The listing builds one solid part. Answer for the finished solid, in the listing's coordinates (mm). A direction names the side the tool comes from. Give positions to 0.01 mm unless a question says otherwise; leave off trailing zeros. Write each loop counter-clockwise with the first axis right and the second up, starting at its lowest first coordinate (ties: lowest second). Pieces come first, ordered by that corner, then holes. Notation, with made-up numbers: (33.25, 12) -> (79.25, 12) arc R26 cw to (79.25, 44) -> close; hole circle Ø10 at (76.25, 57.25). An arc over 180 degrees is marked (long way). Use CSV: the item, a comma, the result in double quotes. Start each with the question number.
from build123d import *

# Parameters (mm, degrees)
SKETCH1_W           = 114.3
SKETCH1_H           = 177.8
SKETCH1_W_2         = 101.6
SKETCH1_H_2         = 165.1
BOSS_EXTRUDE1_DEPTH = 4.7625
SKETCH2_W           = 12.38677804
SKETCH2_H           = 4.7625
SKETCH2_W_2         = 12.7
BOSS_EXTRUDE2_DEPTH = 4.7625
SKETCH3_W           = 12.7
SKETCH3_H           = 4.7625
BOSS_EXTRUDE3_DEPTH = 4.7625
SKETCH4_W           = 12.7
SKETCH4_H           = 177.8
SKETCH4_W_2         = 3.81
SKETCH4_H_2         = 127
BOSS_EXTRUDE4_DEPTH = 4.7625
FILLET1_R           = 1.905


with BuildPart() as part:
    # Sketch1 → Boss-Extrude1 (new body)
    with BuildSketch(Plane(origin=(0, 0, 0), x_dir=(1, 0, 0), z_dir=(0, 1, 0))):
        Rectangle(SKETCH1_W, SKETCH1_H)
        Rectangle(SKETCH1_W_2, SKETCH1_H_2, mode=Mode.SUBTRACT)
    extrude(amount=BOSS_EXTRUDE1_DEPTH)

    # Sketch2 → Boss-Extrude2 (add)
    with BuildSketch(Plane.XY.offset(88.9)):
        with Locations((-38.1, 2.38125)):
            Rectangle(SKETCH2_W, SKETCH2_H)
        with Locations((12.7, 2.38125)):
            Rectangle(SKETCH2_W_2, SKETCH2_H)
    extrude(amount=BOSS_EXTRUDE2_DEPTH)

    # Sketch3 → Boss-Extrude3 (add)
    with BuildSketch(Plane(origin=(0, 0, -88.9), x_dir=(-1, 0, 0), z_dir=(0, 0, -1))):
        with Locations((-38.1, 2.38125)):
            Rectangle(SKETCH3_W, SKETCH3_H)
        with Locations((12.7, 2.38125)):
            Rectangle(SKETCH3_W, SKETCH3_H)
    extrude(amount=BOSS_EXTRUDE3_DEPTH)

    # Sketch4 → Boss-Extrude4 (add)
    # profile 1 of 2: a face of its own
    with BuildSketch(Plane(origin=(0, 4.7625, 0), x_dir=(-1, 0, 0), z_dir=(0, 1, 0))):
        with Locations((12.7, 0)):
            Rectangle(SKETCH4_W, SKETCH4_H)
        with Locations((12.7, 0)):
            Rectangle(SKETCH4_W_2, SKETCH4_H_2, mode=Mode.SUBTRACT)
    # profile 2 of 2: a face of its own
    with BuildSketch(Plane(origin=(0, 4.7625, 0), x_dir=(-1, 0, 0), z_dir=(0, 1, 0))):
        with Locations((-12.7, 0)):
            Rectangle(SKETCH4_W, SKETCH4_H)
        with Locations((-12.7, 0)):
            Rectangle(SKETCH4_W_2, SKETCH4_H_2, mode=Mode.SUBTRACT)
    extrude(amount=-BOSS_EXTRUDE4_DEPTH)

    # Fillet1
    fillet1_edges = [part.edges().sort_by_distance(p)[0] for p in [
        (-10.795, 2.38125, -63.5),
        (-14.605, 2.38125, -63.5),
        (10.795, 2.38125, -63.5),
        (14.605, 2.38125, -63.5),
        (-10.795, 2.38125, 63.5),
        (-14.605, 2.38125, 63.5),
        (10.795, 2.38125, 63.5),
        (14.605, 2.38125, 63.5),
        (-6.35, 2.38125, 82.55),
        (6.35, 2.38125, 82.55),
        (-6.35, 2.38125, -82.55),
        (6.35, 2.38125, -82.55),
        (-19.05, 2.38125, -82.55),
        (-50.8, 2.38125, -82.55),
        (-50.8, 2.38125, 82.55),
        (-19.05, 2.38125, 82.55),
        (19.05, 2.38125, 82.55),
        (50.8, 2.38125, 82.55),
        (19.05, 2.38125, -82.55),
        (50.8, 2.38125, -82.55),
    ]]
    fillet(fillet1_edges, radius=FILLET1_R - 0.0001)  # a hair under: the kernel refuses the full size


solid = part.part
Q1. Straight lines are drawn through the part: L1, parallel to X at y = 0.7, z = 61 (3 decimals); L2, parallel to X at y = 4.25, z = -72.5; L3, parallel to Z at x = -3, y = 2.45. For each, find the intervals that lie inside material, in ascending order.
Q2. Section B-B on z = -58 is taken. State how many separate pieces and enclosed holes the cut face has, then the cut area to 3 significant figures.
Q3. Section D-D on x = 41 is taken. Give the vertices of the cut face in (y, z), then the cut area to 3 significant figures.
Q4. For faces 1 (the face through (6.35, 2, -1)), 2 (the face through (-44.293, 2, 91)), 3 (the face through (-38, 2, -88.9)), 4 (the face through (44.45, 2, -91)), 5 (the face through (31.75, 2, -91)), determine the directions among +Z, -Z, +X, -X, +Y, -Y from which every point of the face is accessible in a straight line to the end or side of a thin tool.
Q5. Section A-A on x = 24 is taken. Give the vertices of the cut face in (y, z).
Q6. Section C-C on z = 68 is taken. Give the vertices of the cut face in (x, y), then the cut area to 3 significant figures.
Q7. Flat-ended cylindrical pins translate along their axes: pin 1 Ø1.4 at (y, z) = (3.5, 91.5) entering from -X; pin 2 Ø2.5 at (y, z) = (2.5, 91.5) entering from +X; pin 3 Ø1.4 at (x, y) = (29.5, 2.5) entering from +Z. Find the tip coordinate at first contact, or state that the pin passes through.
Output:
1,L1,"-57.15 to -50.8, -19.05 to -14.605, -10.795 to -6.35, 6.35 to 10.795, 14.605 to 19.05, 50.8 to 57.15"
1,L2,"-57.15 to -50.8, -19.05 to -6.35, 6.35 to 19.05, 50.8 to 57.15"
1,L3,"-88.9 to -82.55, 82.55 to 88.9"
2,separate pieces,"6"
2,enclosed holes,"0"
2,area,"145 mm²"
3,outline,"(0, -93.66) -> (4.76, -93.66) -> (4.76, -82.55) -> (0, -82.55) -> close; (0, 82.55) -> (4.76, 82.55) -> (4.76, 88.9) -> (0, 88.9) -> close"
3,area,"83.2 mm²"
4,face 1,"+Y, -Y"
4,face 2,"+Z, -X, +Y, -Y"
4,face 3,"-Z, -X, +Y, -Y"
4,face 4,"-Z, +X, +Y, -Y"
4,face 5,"-Z, +Y, -Y"
5,outline,"(0, -88.9) -> (4.76, -88.9) -> (4.76, -82.55) -> (0, -82.55) -> close; (0, 82.55) -> (4.76, 82.55) -> (4.76, 88.9) -> (0, 88.9) -> close"
6,outline,"(-57.15, 0) -> (-50.8, 0) -> (-50.8, 4.76) -> (-57.15, 4.76) -> close; (-19.05, 0) -> (-6.35, 0) -> (-6.35, 4.76) -> (-19.05, 4.76) -> close; (6.35, 0) -> (19.05, 0) -> (19.05, 4.76) -> (6.35, 4.76) -> close; (50.8, 0) -> (57.15, 0) -> (57.15, 4.76) -> (50.8, 4.76) -> close"
6,area,"181 mm²"
7,pin 1,"x = -44.29"
7,pin 2,"x = 19.05"
7,pin 3,"z = 88.9"
